Part print with two shaded views. Sizes in mm from the minimum x, y, z corner. A direction names the side the tool comes from. Coordinates: 2 decimals unless noted, no trailing zeros. One line per item, written item: value. Start each with the question number.
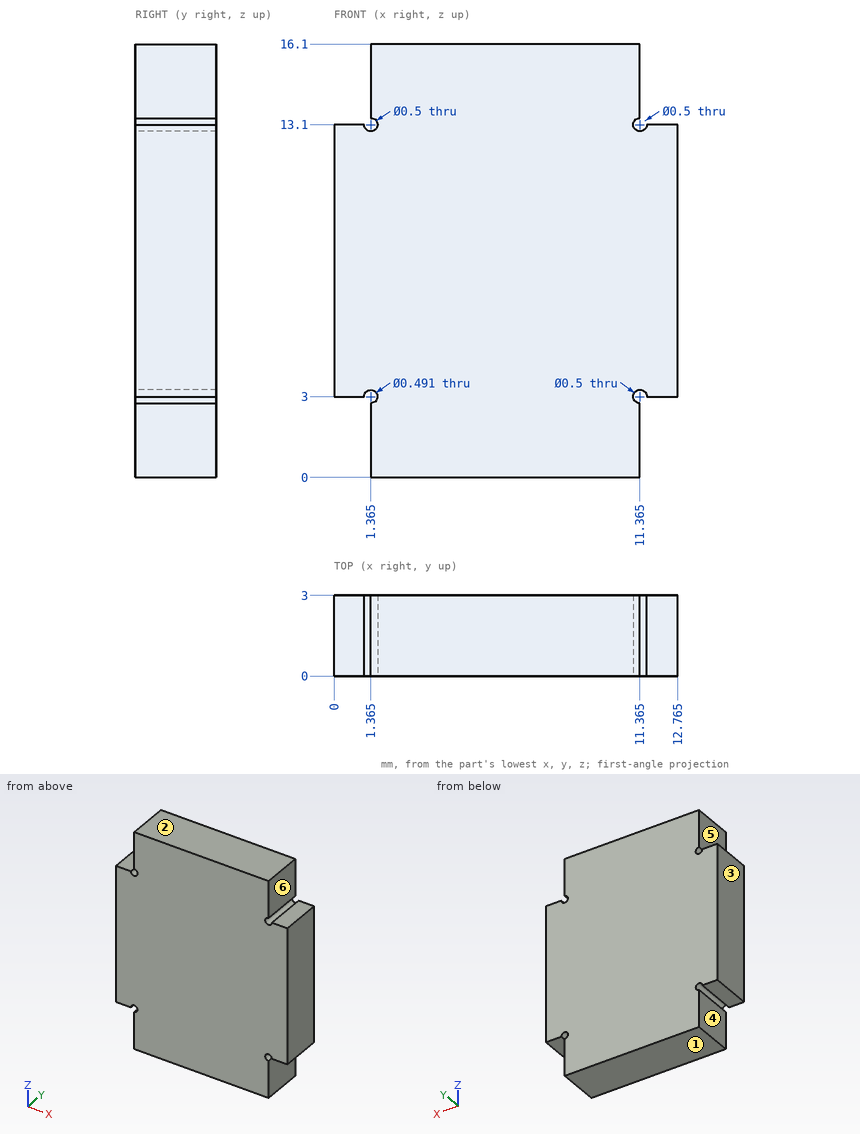
Item 1: Drop flat-ended pins along their axis: pin 1 Ø0.9 at (x, y) = (0.5, 2) entering from +Z; pin 2 Ø0.9 at (x, y) = (12, 1) entering from -Z; pin 3 Ø1.4 at (y, z) = (1.5, 15) entering from +X (1 decimal). Give the stop position or say it passes through.
Item 2: Two-plate mould, pull along Z, no slides. Class the marked faces 1, 2 and 3: +Z half, -Z half, draft (parallel to the pull), parting line (faces both ways), or undercut.
Item 3: Probe probe 1 along Z at (x, y) = (0.5, 0.65); probe 2 along X at (y, z) = (2.35, 14) (1 decimal). List the from-to ranges inside material, lowest first.
Item 4: Tool access for the marked faces 4, 5 and 6: list every direction of +Z, -Z, +X, -X, +Y, -Y with a clear straight run to the whole face (end or side of a thin tool).
Worked out:
1. pin 1: stops at z = 13.1
1. pin 2: stops at z = 3
1. pin 3: stops at x = 11.4
2. face 1: -Z half
2. face 2: +Z half
2. face 3: draft
3. probe 1: z = 3 to 13.1
3. probe 2: x = 1.4 to 11.4
4. face 4: -Z, -X, +Y, -Y
4. face 5: +Z, -X, +Y, -Y
4. face 6: +Z, +X, +Y, -Y
